Part model, mm, in its own coordinate system. A direction names the side the tool comes from. Round coordinates to 2 decimals unless told otherwise and drop trailing zeros. Loops run counter-clockwise (first coordinate to the right, second up) from the corner with the lowest first, then second, coordinate; pieces in that order, holes last.
1) 3-axis set-ups, long thin cutter, end or side, ignore diameter. For faces 4 (the flat face through (4, 61, -28)), 5 (the flat face through (4, 59, 0)), 6 (the cylindrical face through (4.563, 0.526, -15.669)): which of +Z, -Z, +X, -X, +Y, -Y reach the whole face in a straight line?
2) Band-saw the part on A-A, the plane z = -25. Write the cut outline in (x, y), then the cut area to 3 significant figures.
3) Band-saw the part on B-B, the plane x = 3.75. Write the cut outline in (y, z).
4) Band-saw the part on C-C, the plane z = -32. Write the cut outline in (x, y).
5) Mould opens along Y. For faces 1 (the flat face through (9, 79, -14)), 2 (the cylindrical face through (4.44, 170.07, -13.02)), 3 (the cylindrical face through (4.563, 164.007, -11.253)) say: +Y half, -Y half, draft (parallel to the pull), parting line (faces both ways), or undercut.
6) Band-saw the part on D-D, the plane y = 85. Write the cut outline in (x, z), then the cut area to 3 significant figures.
7) Probe line 1 (Z direction, x = 8, y = 137.5); line 2 (Z direction, x = 6.5, y = 148); line 3 (Z direction, x = 5, y = 46.5). List the from-to ranges inside material, lowest first.
8) Drop flat-ended pins along their axis: P1, Ø3, axis at x = 6.5, z = -11.5, coming from the -Y side; P2, Ø2, axis at x = 5.5, y = 48, coming from the +Z side; P3, Ø2, axis at x = 1.5, z = 4, coming from the -Y side. Give the stop position or say it passes through.
from build123d import *

# Parameters (mm, degrees)
EXTRUDE_6_DEPTH      = 9
SKETCH_8_R           = 23.25
CUT_EXTRUDE_6_DEPTH  = 7
SKETCH_9_R           = 19.25
CUT_EXTRUDE_7_DEPTH  = 7
SKETCH_13_R          = 23.25
EXTRUDE_9_DEPTH      = 9
SKETCH_14_R          = 21.1
CUT_EXTRUDE_8_DEPTH  = 10
SKETCH_26_R          = 1.75
CUT_EXTRUDE_14_DEPTH = 10
SKETCH_25_R          = 1.25
CUT_EXTRUDE_15_DEPTH = 10


with BuildPart() as part:
    # 草图1 → 凸台-拉伸6 (new body)
    with BuildSketch(Plane(origin=(0, 0, 0), x_dir=(0, 0, -1), z_dir=(1, 0, 0))):
        with BuildLine():
            Line((0, 0), (0, 120))
            ThreePointArc((0, 120), (14, 170.086792761), (28, 120))
            Line((28, 120), (28, 0))
            ThreePointArc((28, 0), (14, -14), (0, 0))
        make_face()
    extrude(amount=EXTRUDE_6_DEPTH)

    # 草图8 → 切除-拉伸6 (cut)
    with BuildSketch(Plane(origin=(9, 0, 0), x_dir=(0, 0, -1), z_dir=(1, 0, 0))):
        with Locations((14, 143.086792761)):
            Circle(SKETCH_8_R)
    extrude(amount=-CUT_EXTRUDE_6_DEPTH, mode=Mode.SUBTRACT)

    # 草图9 → 切除-拉伸7 (cut)
    with BuildSketch(Plane(origin=(2, 0, 0), x_dir=(0, 0, -1), z_dir=(1, 0, 0))):
        with Locations((14, 143.086792761)):
            Circle(SKETCH_9_R)
    extrude(amount=-CUT_EXTRUDE_7_DEPTH, mode=Mode.SUBTRACT)

    # 草图13 → 凸台-拉伸9 (add)
    with BuildSketch(Plane(origin=(9, 0, 0), x_dir=(0, 0, -1), z_dir=(1, 0, 0))):
        with Locations((14, 143.086792761)):
            Circle(SKETCH_13_R)
    extrude(amount=-EXTRUDE_9_DEPTH)

    # 草图14 → 切除-拉伸8 (cut)
    with BuildSketch(Plane(origin=(9, 0, 0), x_dir=(0, 0, -1), z_dir=(1, 0, 0))):
        with Locations((14, 143.086792761)):
            Circle(SKETCH_14_R)
    extrude(amount=-CUT_EXTRUDE_8_DEPTH, mode=Mode.SUBTRACT)

    # 草图26 → 切除-拉伸14 (cut)
    with BuildSketch(Plane(origin=(9, 0, 0), x_dir=(0, 0, -1), z_dir=(1, 0, 0))):
        with Locations((14, 0)):
            Circle(SKETCH_26_R)
    extrude(amount=-CUT_EXTRUDE_14_DEPTH, mode=Mode.SUBTRACT)

    # 草图25 → 切除-拉伸15 (cut)
    with BuildSketch(Plane.ZY):
        with Locations((9.2, 143.086792761)):
            Circle(SKETCH_25_R)
        with Locations((-14, 119.886792761)):
            Circle(SKETCH_25_R)
        with Locations((-37.2, 143.086792761)):
            Circle(SKETCH_25_R)
        with Locations((-14, 166.286792761)):
            Circle(SKETCH_25_R)
    extrude(amount=-CUT_EXTRUDE_15_DEPTH, mode=Mode.SUBTRACT)


solid = part.part
Reported:
1. face 4: -Z, +X, -X, -Y
1. face 5: +Z, +X, -X, -Y
1. face 6: +X, -X
2. outline: (0, -8.66) - (9, -8.66) - (9, 125.08) - (0, 125.08) - close; (0, 161.09) - (9, 161.09) - (9, 167.74) - (0, 167.74) - close
2. area: 1,260 mm2
3. outline: (0, -28) - (120, -28) arc R27 ccw (long way) to (120, 0) - (0, 0) arc R14 ccw to start; hole circle Ø3.5 at (0, -14); hole circle Ø2.5 at (119.89, -14); hole circle Ø42.2 at (143.09, -14); hole circle Ø2.5 at (143.09, -37.2); hole circle Ø2.5 at (143.09, 9.2); hole circle Ø2.5 at (166.29, -14)
4. outline: (0, 122.96) - (9, 122.96) - (9, 132.08) - (0, 132.08) - close; (0, 154.1) - (9, 154.1) - (9, 163.21) - (0, 163.21) - close
5. face 1: draft
5. face 2: parting line
5. face 3: undercut
6. outline: (0, -28) - (9, -28) - (9, 0) - (0, 0) - close
6. area: 252 mm2
7. line 1: z = -40.42 to -34.35, 6.35 to 12.42
7. line 2: z = -40.55 to -34.52, 6.52 to 12.55
7. line 3: z = -28 to 0
8. P1: stops at y = -13.96
8. P2: stops at z = 0
8. P3: stops at y = 122.11
